```python
from build123d import *

# Parameters (mm, degrees)
SKETCH1_R           = 7.9375
SKETCH1_R_2         = 2.413
SKETCH1_R_3         = 3.175
SKETCH1_R_4         = 3.429
BOSS_EXTRUDE1_DEPTH = 7.62
SKETCH2_R           = 7.9375
SKETCH2_R_2         = 3.81
BOSS_EXTRUDE2_DEPTH = 2.54
SKETCH3_W           = 154.94
SKETCH3_H           = 11.43
BOSS_EXTRUDE3_DEPTH = 15.24
FILLET1_R           = 5.08
SKETCH5_R           = 2.286
CUT_EXTRUDE1_DEPTH  = 128
CUT_EXTRUDE2_DEPTH  = 6.35
CUT_EXTRUDE3_DEPTH  = 6.35


with BuildPart() as part:
    # Sketch1 → Boss-Extrude1 (new body)
    with BuildSketch(Plane(origin=(0, 0, 0), x_dir=(0, 0, -1), z_dir=(1, 0, 0))):
        with BuildLine():
            Line((0, 0), (127, 0))
            Line((127, 0), (100.900837488, 6.993249518))
            ThreePointArc((100.900837488, 6.993249518), (97.889599245, 8.807630529), (96.305117976, 11.94593474))
            Line((96.305117976, 11.94593474), (96.305117976, 25.91593474))
            ThreePointArc((96.305117976, 25.91593474), (94.817220425, 29.508037188), (91.225117976, 30.99593474))
            Line((91.225117976, 30.99593474), (40.425117976, 30.99593474))
            ThreePointArc((40.425117976, 30.99593474), (36.833015528, 29.508037188), (35.345117976, 25.91593474))
            Line((35.345117976, 25.91593474), (35.345117976, 16.51))
            ThreePointArc((35.345117976, 16.51), (33.857220425, 12.917897552), (30.265117976, 11.43))
            Line((30.265117976, 11.43), (0, 11.43))
            Line((0, 11.43), (-20.139487758, 11.43))
            Line((-20.139487758, 11.43), (-33.393348427, 24.683860669))
            ThreePointArc((-33.393348427, 24.683860669), (-34.855521636, 27.76537759), (-34.039193709, 31.077069869))
            ThreePointArc((-34.039193709, 31.077069869), (-35.088692293, 41.466034818), (-45.477657242, 42.515533402))
            ThreePointArc((-45.477657242, 42.515533402), (-48.789349521, 41.699205475), (-51.870866442, 43.161378684))
            Line((-51.870866442, 43.161378684), (-53.208352597, 44.49886484))
            ThreePointArc((-53.208352597, 44.49886484), (-53.705674947, 45.203111295), (-53.938776392, 46.033145213))
            ThreePointArc((-53.938776392, 46.033145213), (-56.302994281, 51.089129932), (-61.291601771, 53.592388411))
            ThreePointArc((-61.291601771, 53.592388411), (-62.869694805, 54.435936137), (-63.5, 56.110649769))
            Line((-63.5, 56.110649769), (-63.5, 127))
            Line((-63.5, 127), (-88.9, 127))
            Line((-88.9, 127), (-88.9, 64.149284844))
            ThreePointArc((-88.9, 64.149284844), (-89.255767512, 62.281658704), (-90.273239134, 60.675623392))
            ThreePointArc((-90.273239134, 60.675623392), (-92.64207664, 54.683557387), (-90.273239134, 48.691491383))
            ThreePointArc((-90.273239134, 48.691491383), (-89.255767512, 47.085456071), (-88.9, 45.217829931))
            Line((-88.9, 45.217829931), (-88.9, 0))
            Line((-88.9, 0), (0, 0))
        make_face()
        with Locations((83.514716058, 9.525)):
            Circle(SKETCH1_R, mode=Mode.SUBTRACT)
        with Locations((-76.2, 114.3)):
            Circle(SKETCH1_R_2, mode=Mode.SUBTRACT)
        with Locations((-76.2, 88.9)):
            Circle(SKETCH1_R_2, mode=Mode.SUBTRACT)
        with Locations((-76.2, 101.6)):
            Circle(SKETCH1_R_2, mode=Mode.SUBTRACT)
        with Locations((-76.2, 76.2)):
            Circle(SKETCH1_R_2, mode=Mode.SUBTRACT)
        with Locations((65.671256734, 22.86)):
            Circle(SKETCH1_R_3, mode=Mode.SUBTRACT)
        with Locations((-62.402467706, 45.156212864)):
            Circle(SKETCH1_R_4, mode=Mode.SUBTRACT)
        with Locations((42.176256734, 22.86)):
            Circle(SKETCH1_R_2, mode=Mode.SUBTRACT)
        with Locations((89.166256734, 22.86)):
            Circle(SKETCH1_R_2, mode=Mode.SUBTRACT)
        with Locations((-83.87907664, 54.683557387)):
            Circle(SKETCH1_R_2, mode=Mode.SUBTRACT)
        with Locations((-40.925858771, 35.62886834)):
            Circle(SKETCH1_R_2, mode=Mode.SUBTRACT)
        Polygon((-63.5, 11.43), (-63.5, 36.83), (-38.1, 11.43), align=None, mode=Mode.SUBTRACT)
    extrude(amount=BOSS_EXTRUDE1_DEPTH)

    # Sketch2 → Boss-Extrude2 (add)
    with BuildSketch(Plane(origin=(7.62, 0, 0), x_dir=(0, 0, -1), z_dir=(1, 0, 0))):
        with Locations((83.514716058, 9.525)):
            Circle(SKETCH2_R)
        with Locations((83.514716058, 9.525)):
            Circle(SKETCH2_R_2, mode=Mode.SUBTRACT)
    extrude(amount=-BOSS_EXTRUDE2_DEPTH)

    # Sketch3 → Boss-Extrude3 (add)
    with BuildSketch(Plane.ZY):
        with Locations((11.43, 5.715)):
            Rectangle(SKETCH3_W, SKETCH3_H)
    extrude(amount=BOSS_EXTRUDE3_DEPTH)

    # Fillet1
    fillet1_edges = [part.edges().sort_by_distance(p)[0] for p in [
        (0, 5.715, -66.04),
    ]]
    fillet(fillet1_edges, radius=FILLET1_R)

    # Sketch5 → Cut-Extrude1 (cut, through all)
    with BuildSketch(Plane.XZ):
        with Locations((-3.81, -50.8)):
            Circle(SKETCH5_R)
        with Locations((-3.81, 0)):
            Circle(SKETCH5_R)
    extrude(amount=-CUT_EXTRUDE1_DEPTH, mode=Mode.SUBTRACT)

    # Sketch6 → Cut-Extrude2 (cut)
    with BuildSketch(Plane.XZ):
        Polygon((1.61593783, -50.8), (-1.097031085, -46.101), (-6.522968915, -46.101), (-9.23593783, -50.8), (-6.522968915, -55.499), (-1.097031085, -55.499), align=None)
        Polygon((-1.097031085, -4.699), (1.61593783, 0), (-1.097031085, 4.699), (-6.522968915, 4.699), (-9.23593783, 0), (-6.522968915, -4.699), align=None)
    extrude(amount=-CUT_EXTRUDE2_DEPTH, mode=Mode.SUBTRACT)

    # Sketch7 → Cut-Extrude3 (cut)
    with BuildSketch(Plane.ZY):
        Polygon((-84.467256734, 25.572968915), (-89.166256734, 28.28593783), (-93.865256734, 25.572968915), (-93.865256734, 20.147031085), (-89.166256734, 17.43406217), (-84.467256734, 20.147031085), align=None)
        Polygon((-37.477256734, 25.572968915), (-42.176256734, 28.28593783), (-46.875256734, 25.572968915), (-46.875256734, 20.147031085), (-42.176256734, 17.43406217), (-37.477256734, 20.147031085), align=None)
        Polygon((45.624858771, 38.341837255), (40.925858771, 41.054806169), (36.226858771, 38.341837255), (36.226858771, 32.915899425), (40.925858771, 30.20293051), (45.624858771, 32.915899425), align=None)
        Polygon((88.57807664, 57.396526302), (83.87907664, 60.109495217), (79.18007664, 57.396526302), (79.18007664, 51.970588472), (83.87907664, 49.257619558), (88.57807664, 51.970588472), align=None)
    extrude(amount=-CUT_EXTRUDE3_DEPTH, mode=Mode.SUBTRACT)


solid = part.part
```
The listing builds one solid part. Answer for the finished solid, in the listing's coordinates (mm). A direction names the side the tool comes from. Give positions to 0.01 mm unless a question says otherwise; leave off trailing zeros. Order: outer loops, then holes, each group sorted by start corner. A loop starts at its lowest first (then second) coordinate and runs counter-clockwise, first axis right, second up. Notation, with made-up numbers: (-30, -30) - (-1, -30) arc R29 cw to (-1, -5) - close; hole circle Ø8 at (51.5, 5.5). An arc over 180 degrees is marked (long way). Answer in a Markdown table with one row per item. Add a question column.
Q1. The part is cut by section C-C (x = -12). Determine the outline of the cut face in (y, z), then the cut area to 3 significant figures.
Q2. Which of the six approach directions +Z, -Z, +X, -X, +Y, -Y give full straight-line access (tool end or side, diameter ignored) to faces 4 (the flat face through (4, 96, 88.9)), 5 (the flat face through (3.76, 24.31, 50.98)), 6 (the flat face through (3.131, 58.734, 86.261))?
Q3. Find the intervals of material crossed by line 1 along Y through (x, z) = (3.5, 76.2); line 2 along Z through (x, y) = (4.5, 43); line 3 along Z through (x, y) = (5, 20.5), in increasing order. Write a range as [from, to].
Q4. For a pull along Z with two mould halves and no side action, classify faces 1 (the flat face through (4, 19, -96.305)), 2 (the flat face through (3.13, 26.91, -86.78)), 3 (the cylindrical face through (3.76, 54.78, 92.64)) as released by +Z, released by -Z, zero draft, split by the parting line, or undercut.
Q5. The part is cut by section A-A (z = 76.2). Determine the outline of the cut face in (x, y), then the cut area to 3 significant figures.
Q6. Given P1, Ø1.5, axis at x = 2.5, z = -81.5, coming from the +Y side; P2, Ø8, axis at x = -9.5, z = -1.5, coming from the +Y side; P3, Ø1.6, axis at x = 5, y = 22, coming from the +Z side, each flat-ended and moving along its own axis, determine where each tip first touches the part or whether it passes through.
Q7. The part is cut by section B-B (y = 114.3). Determine the outline of the cut face in (x, z).
Determined:
| question | item | result |
|---|---|---|
| 1 | outline | (0, -66.04) - (11.43, -66.04) - (11.43, 88.9) - (0, 88.9) - close |
| 1 | area | 1,770 mm² |
| 2 | face 4 | +Z, +X, -X, +Y |
| 2 | face 5 | +X, -X |
| 2 | face 6 | -X |
| 3 | line 1 | y = [0, 73.79], [78.61, 86.49], [91.31, 99.19], [104.01, 111.89], [116.71, 127] |
| 3 | line 2 | z = [37.21, 44.64], [51.7, 59.74], [65.07, 88.9] |
| 3 | line 3 | z = [-96.31, -93.87], [-84.47, -67.8], [-63.55, -46.88], [-37.48, -35.35], [29.21, 47.17], [63.5, 88.9] |
| 4 | face 1 | released by -Z |
| 4 | face 2 | undercut |
| 4 | face 3 | released by +Z |
| 5 | outline | (-15.24, 0) - (7.62, 0) - (7.62, 73.79) - (0, 73.79) - (0, 11.43) - (-15.24, 11.43) - close; (0, 78.61) - (7.62, 78.61) - (7.62, 86.49) - (0, 86.49) - close; (0, 91.31) - (7.62, 91.31) - (7.62, 99.19) - (0, 99.19) - close; (0, 104.01) - (7.62, 104.01) - (7.62, 111.89) - (0, 111.89) - close; (0, 116.71) - (7.62, 116.71) - (7.62, 127) - (0, 127) - close |
| 5 | area | 995 mm² |
| 6 | P1 | stops at y = 31 |
| 6 | P2 | stops at y = 11.43 |
| 6 | P3 | stops at z = 88.9 |
| 7 | outline | (0, 63.5) - (7.62, 63.5) - (7.62, 73.79) - (0, 73.79) - close; (0, 78.61) - (7.62, 78.61) - (7.62, 88.9) - (0, 88.9) - close |
